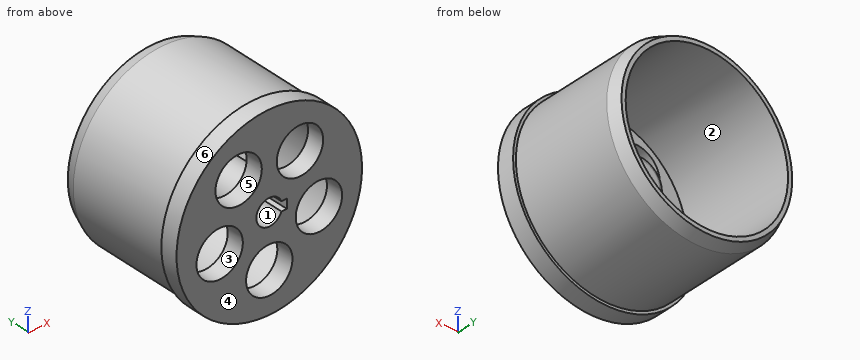
from build123d import *

# Parameters (mm, degrees)
SKETCH1_R           = 50.8
SKETCH1_R_2         = 12.7
BOSS_EXTRUDE1_DEPTH = 9.525
SKETCH2_R           = 49.276
SKETCH2_R_2         = 44.45
BOSS_EXTRUDE2_DEPTH = 63.5
SKETCH3_R           = 12.7
BOSS_EXTRUDE3_DEPTH = 15.875
CHAMFER1_SIZE       = 6.35
CHAMFER1_SIZE2      = 2.54
SKETCH4_R           = 12.7
BOSS_EXTRUDE4_DEPTH = 6.35
FILLET1_R           = 2.54


with BuildPart() as part:
    # Sketch1 → Boss-Extrude1 (new body)
    with BuildSketch(Plane(origin=(0, 0, 0), x_dir=(1, 0, 0), z_dir=(0, 1, 0))):
        Circle(SKETCH1_R)
        with Locations((-16.795963584, -23.117660614)):
            Circle(SKETCH1_R_2, mode=Mode.SUBTRACT)
        with Locations((16.795963584, -23.117660614)):
            Circle(SKETCH1_R_2, mode=Mode.SUBTRACT)
        with BuildLine():
            Line((9.6, -2.5), (6.64529909, -2.5))
            ThreePointArc((6.64529909, -2.5), (-7.1, 0), (6.64529909, 2.5))
            Line((6.64529909, 2.5), (9.6, 2.5))
            Line((9.6, 2.5), (9.6, -2.5))
        make_face(mode=Mode.SUBTRACT)
        with Locations((-27.176439953, 8.830160614)):
            Circle(SKETCH1_R_2, mode=Mode.SUBTRACT)
        with BuildLine():
            ThreePointArc((0, 15.875), (-12.7, 28.575), (0, 41.275))
            ThreePointArc((0, 41.275), (12.7, 28.575), (0, 15.875))
        make_face(mode=Mode.SUBTRACT)
        with Locations((27.176439953, 8.830160614)):
            Circle(SKETCH1_R_2, mode=Mode.SUBTRACT)
    extrude(amount=BOSS_EXTRUDE1_DEPTH)

    # Sketch2 → Boss-Extrude2 (add)
    with BuildSketch(Plane(origin=(0, 9.525, 0), x_dir=(1, 0, 0), z_dir=(0, 1, 0))):
        Circle(SKETCH2_R)
        Circle(SKETCH2_R_2, mode=Mode.SUBTRACT)
    extrude(amount=BOSS_EXTRUDE2_DEPTH)

    # Sketch3 → Boss-Extrude3 (add)
    with BuildSketch(Plane(origin=(0, 9.525, 0), x_dir=(1, 0, 0), z_dir=(0, 1, 0))):
        Circle(SKETCH3_R)
        with BuildLine():
            Line((9.6, -2.5), (6.64529909, -2.5))
            ThreePointArc((6.64529909, -2.5), (-7.1, 0), (6.64529909, 2.5))
            Line((6.64529909, 2.5), (9.6, 2.5))
            Line((9.6, 2.5), (9.6, -2.5))
        make_face(mode=Mode.SUBTRACT)
    extrude(amount=BOSS_EXTRUDE3_DEPTH)

    # Chamfer1
    chamfer1_edges = [part.edges().sort_by_distance(p)[0] for p in [
        (-49.276, 73.025, 0),
    ]]
    chamfer1_side = [part.faces().sort_by_distance(p)[0] for p in [
        (-49.276, 41.275, 0),
    ]]
    chamfer(chamfer1_edges, length=CHAMFER1_SIZE, length2=CHAMFER1_SIZE2, reference=chamfer1_side[0])

    # Sketch4 → Boss-Extrude4 (add)
    with BuildSketch(Plane(origin=(0, 25.4, 0), x_dir=(1, 0, 0), z_dir=(0, 1, 0))):
        Circle(SKETCH4_R)
    extrude(amount=BOSS_EXTRUDE4_DEPTH)

    # Fillet1
    fillet1_edges = [part.edges().sort_by_distance(p)[0] for p in [
        (-12.7, 31.75, 0),
    ]]
    fillet(fillet1_edges, radius=FILLET1_R)


solid = part.part
Work out the finished part from the listing and answer in its coordinate system (mm). Face numbers are marked on the shaded views. A direction names the side the tool comes from. Coordinates: 2 decimals unless noted, no trailing zeros. Write each loop counter-clockwise with the first axis right and the second up, starting at its lowest first coordinate (ties: lowest second). Pieces come first, ordered by that corner, then holes.
1. For a pull along X with two mould halves and no side action, classify the marked faces 4, 5 and 6 as +X half, -X half, draft (parallel to the pull), parting line (faces both ways), or undercut.
Results list:
face 4: draft
face 5: undercut
face 6: parting line
2. The part is cut by section B-B, the plane y = 6. Write down the section's boundary in (x, z) (3 decimals).
Results list:
outline: circle Ø101.6 at (0, 0); hole circle Ø25.4 at (-27.176, -8.83); hole circle Ø25.4 at (-16.796, 23.118); hole circle Ø25.4 at (0, -28.575); hole circle Ø25.4 at (16.796, 23.118); hole (6.645, -2.5) - (9.6, -2.5) - (9.6, 2.5) - (6.645, 2.5) arc R7.1 ccw (long way) to start; hole circle Ø25.4 at (27.176, -8.83)
3. The part is cut by section C-C, the plane z = 0. State how many separate pieces and enclosed holes the cut face has, and give its area (3 significant figures).
Results list:
separate pieces: 3
enclosed holes: 0
area: 1,350 mm2
4. Consider line 1 along X through (y, z) = (17.25, 0); line 2 along Z through (x, y) = (0, 25); line 3 along Z through (x, y) = (0, 58). Determine where each line is inside the solid, lowest interval first.
Results list:
line 1: x = -49.28 to -44.45, -12.7 to -7.1, 9.6 to 12.7, 44.45 to 49.28
line 2: z = -49.28 to -44.45, -12.7 to -7.1, 7.1 to 12.7, 44.45 to 49.28
line 3: z = -49.28 to -44.45, 44.45 to 49.28
5. For the marked faces 1, 2 and 3, determine the directions among +Z, -Z, +X, -X, +Y, -Y from which every point of the face is accessible in a straight line to the end or side of a thin tool.
Results list:
face 1: -Y
face 2: +Y
face 3: +Y, -Y
6. The part is cut by section A-A, the plane x = 0. Write down the section's boundary in (y, z) (3 decimals).
Results list:
outline: (0, -50.8) - (9.525, -50.8) - (9.525, -49.276) - (66.675, -49.276) - (73.025, -46.736) - (73.025, -44.45) - (9.525, -44.45) - (9.525, -41.275) - (0, -41.275) - close; (0, -15.875) - (9.525, -15.875) - (9.525, -12.7) - (29.21, -12.7) arc R2.54 ccw to (31.75, -10.16) - (31.75, 10.16) arc R2.54 ccw to (29.21, 12.7) - (9.525, 12.7) - (9.525, 44.45) - (73.025, 44.45) - (73.025, 46.736) - (66.675, 49.276) - (9.525, 49.276) - (9.525, 50.8) - (0, 50.8) - (0, 7.1) - (25.4, 7.1) - (25.4, -7.1) - (0, -7.1) - close
7. Flat-ended cylindrical pins translate along their axes: pin 1 (3 mm diameter, centred on x = -5.5, z = -8, fed in from +Y); pin 2 (1.5 mm diameter, centred on x = 8.5, y = 14.5, fed in from +Z); pin 3 (5 mm diameter, centred on y = 42.5, z = -28, fed in from -X); pin 4 (11.5 mm diameter, centred on x = 3, z = -0.5, fed in from -Y). Find the tip coordinate at first contact, or state that the pin passes through.
Results list:
pin 1: stops at y = 31.75
pin 2: stops at z = 48.66
pin 3: stops at x = -42.16
pin 4: stops at y = 0
8. The part is cut by section D-D, the plane y = 33.5. Write down the section's boundary in (x, z), and give its area (3 significant figures).
Results list:
outline: circle Ø98.55 at (0, 0); hole circle Ø88.9 at (0, 0)
area: 1,420 mm2
